Here's how the part is built. I have some questions about the finished solid (model axes, mm). Round coordinates to 2 decimals unless told otherwise and drop trailing zeros. Write each loop counter-clockwise with the first axis right and the second up, starting at its lowest first coordinate (ties: lowest second). Pieces come first, ordered by that corner, then holes. Notation, with made-up numbers: (64.5, 9) - (94.5, 9) arc R24 cw to (94.5, 41) - close; hole circle Ø9 at (21.25, 53.5). An arc over 180 degrees is marked (long way). Write item = value, one per line. Start each with the question number.
Item 1: If I drill on line 1 along Z through (x, y) = (26, -10.5); line 2 along Z through (x, y) = (25.4, -23) (3 decimals); line 3 along X through (y, z) = (-6, 307.29), over which ranges is the centre line in solid material (lowest first)? Write a range as [from, to].
Item 2: If we section it at B-B (z = 307.29): Please give me the cut outline in (x, y) (3 decimals), and give its area (3 significant figures).
Item 3: If we section it at C-C (y = -21.75): Please give me the cut outline in (x, z) (3 decimals).
Item 4: For P1, Ø10, axis at x = 63.5, z = 12.7, coming from the -Y side; P2, Ø5, axis at y = -12.7, z = 380, coming from the -X side, each with a flat end and sliding along its axis, tell me the tip position at first contact or that it passes through.
Item 5: If we section it at A-A (x = 63.5): Please give me the cut outline in (y, z) (3 decimals).
```python
from build123d import *

# Parameters (mm, degrees)
F1_DEPTH       = 25.4
F3_D           = 8.5
F3_DEPTH       = 23.9
F3_TIP         = 2.5536576309
F5_D           = 8.8
F5_CBORE_D     = 14.25
F5_CBORE_DEPTH = 8
F7_D           = 11
F7_CBORE_D     = 17.25
F7_CBORE_DEPTH = 10


with BuildPart() as f1:
    # F0 (on Front) → F1 (new body)
    with BuildSketch(Plane.XZ):
        Polygon((0, 400), (0, 0), (76.2, 0), (76.2, 355.6), (50.8, 400), align=None)
    extrude(amount=F1_DEPTH)

    # F3
    with Locations(Plane(origin=(0, 0, 0), x_dir=(0, -1, 0), z_dir=(-1, 0, 0))):
        with Locations((12.7, 20), (12.7, 380)):
            Hole(F3_D / 2, depth=F3_DEPTH)
            with Locations((0, 0, -(F3_DEPTH + F3_TIP / 2))):  # 118° drill point
                Cone(0, F3_D / 2, F3_TIP, mode=Mode.SUBTRACT)

    # F5 (through all)
    with Locations(Plane.XZ.offset(25.4)):
        with Locations((38.1, 12.7), (63.5, 12.7)):
            CounterBoreHole(F5_D / 2, F5_CBORE_D / 2, F5_CBORE_DEPTH)

    # F7 (through all)
    with Locations(Plane.XZ.offset(25.4)):
        with Locations((25.4, 340.31), (25.4, 307.29)):
            CounterBoreHole(F7_D / 2, F7_CBORE_D / 2, F7_CBORE_DEPTH)


solid = f1.part
```
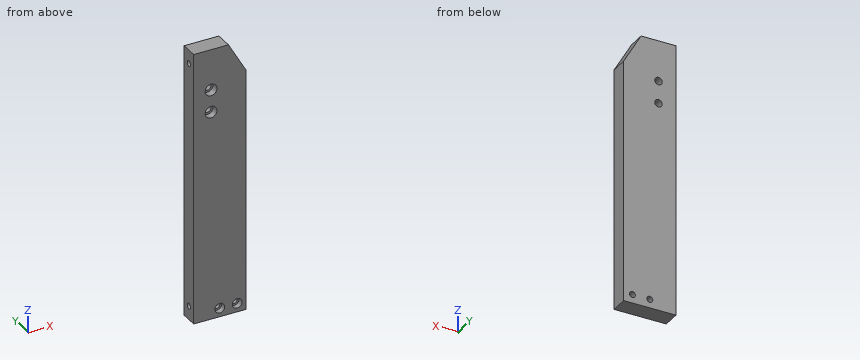
Reply:
q1.line_1 = [0, 301.82], [312.76, 334.84], [345.78, 400]
q1.line_2 = [0, 298.665], [315.915, 331.685], [348.935, 400]
q1.line_3 = [0, 19.9], [30.9, 76.2]
q2.outline = (0, -25.4) - (16.775, -25.4) - (16.775, -15.4) - (19.9, -15.4) - (19.9, 0) - (0, 0) - close; (30.9, -15.4) - (34.025, -15.4) - (34.025, -25.4) - (76.2, -25.4) - (76.2, 0) - (30.9, 0) - close
q2.area = 1,590 mm2
q3.outline = (0, 0) - (76.2, 0) - (76.2, 355.6) - (50.8, 400) - (0, 400) - close; hole circle Ø17.25 at (25.4, 307.29); hole circle Ø17.25 at (25.4, 340.31); hole circle Ø14.25 at (38.1, 12.7); hole circle Ø14.25 at (63.5, 12.7)
q4.P1 = -17.4
q4.P2 = 24.95
q5.outline = (-25.4, 0) - (0, 0) - (0, 8.3) - (-17.4, 8.3) - (-17.4, 5.575) - (-25.4, 5.575) - close; (-25.4, 19.825) - (-17.4, 19.825) - (-17.4, 17.1) - (0, 17.1) - (0, 377.8) - (-25.4, 377.8) - close
